Check sheet for the modelled part. Datum: model origin and axes. Units: mm. Give positions to 0.01 mm unless a question says otherwise; leave off trailing zeros. Order: outer loops, then holes, each group sorted by start corner. A loop starts at its lowest first (then second) coordinate and runs counter-clockwise, first axis right, second up.
Autodesk Inventor part; units mm, degrees
ref_plane "YZ Plane" through (0, 0, 0) normal (1, 0, 0) x (0, 1, 0)
ref_plane "XZ Plane" through (0, 0, 0) normal (0, 1, 0) x (-1, 0, 0)
ref_plane "XY Plane" through (0, 0, 0) normal (0, 0, 1) x (1, 0, 0)
sketch "Skizze1" plane through (0, 0, 0) normal (0, 0, 1) x (1, 0, 0)
  line L0 (-4.9, 0) -> (4.9, 0)
  line L1 (0, -1.8) -> (0, 10.8)
  line L2 (3.5, 9) -> (3.5, 3)
  line L3 (3.5, 3) -> (-3.5, 3)
  line L4 (-3.5, 3) -> (-3.5, 9)
  line L5 (-1.5, 9) -> (0, 7.5)
  line L6 (0, 7.5) -> (1.5, 9)
  line L7 (-3.5, 9) -> (-1.5, 9)
  line L8 (1.5, 9) -> (3.5, 9)
  circle A0 centre (0, 7.8536) radius 0.25
  point P0 (0, 0)
  dimension "d0" = 6
  dimension "d1" = 18
  dimension "d2" = 7
  dimension "d3" = 90
  dimension "d4" = 15
  dimension "d9" = 0.5
  dimension "d10" = 15.7071
revolve "Umdrehung1" add sketch "Skizze1" angle 360 about axis through (-10, 0, 0) along (1, 0, 0) contours L3 L4 L7 L5 L1 | L1 L6 L8 L2 L3
chamfer "Fase1" distance 0.5 angle 45 2 edges at (-3.5, -9, 0) (3.5, -9, 0)
properties part number "13_0204_044"
Q1. Sectioned sample at A-A, the plane y = 0. Record the cut outline in (x, z).
Q2. Material ranges on line 1 (Y direction, x = -2.5, z = 1.25); line 2 (Z direction, x = 0.75, y = 0); line 3 (X direction, y = -5.25, z = 6), recorded low to high.
Q3. Sectioned sample at C-C, the plane x = 2. Record the cut outline in (y, z), plus the area to 3 significant figures.
Q4. Sectioned sample at D-D, the plane x = 0.75. Record the cut outline in (y, z).
Q5. Go/stop test with flat-tipped pins: P1, Ø3.5, axis at y = 0, z = 0, coming from the +X side; P2, Ø3, axis at x = 2.5, z = -3.5, coming from the +Y side. Record where each tip stops, or that it passes through.
Filled in:
1. outline: (-3.5, -8.5) - (-3, -9) - (-1.5, -9) - (0, -7.5) - (1.5, -9) - (3, -9) - (3.5, -8.5) - (3.5, -3) - (-3.5, -3) - close; (-3.5, 3) - (3.5, 3) - (3.5, 8.5) - (3, 9) - (1.5, 9) - (0, 7.5) - (-1.5, 9) - (-3, 9) - (-3.5, 8.5) - close
2. line 1: y = -8.91 to -2.73, 2.73 to 8.91
2. line 2: z = -8.25 to -3, 3 to 8.25
2. line 3: x = -3.5 to -0.47, 0.47 to 3.5
3. outline: circle Ø18 at (0, 0); hole circle Ø6 at (0, 0)
3. area: 226 mm2
4. outline: circle Ø16.5 at (0, 0); hole circle Ø6 at (0, 0)
5. P1: passes through
5. P2: stops at y = 8.77
